Model file for the job. Use its own axes, mm. Face numbers are marked on the shaded views. A direction names the side the tool comes from. Coordinates: 2 decimals unless noted, no trailing zeros. Write each loop counter-clockwise with the first axis right and the second up, starting at its lowest first coordinate (ties: lowest second). Pieces come first, ordered by that corner, then holes. Notation, with made-up numbers: (4, 31.5) -> (8, 31.5) arc R36 cw to (8, 66.5) -> close; hole circle Ø6 at (41, 73.5). An arc over 180 degrees is marked (long way). Write item = value, one per line. Start each with the question number.
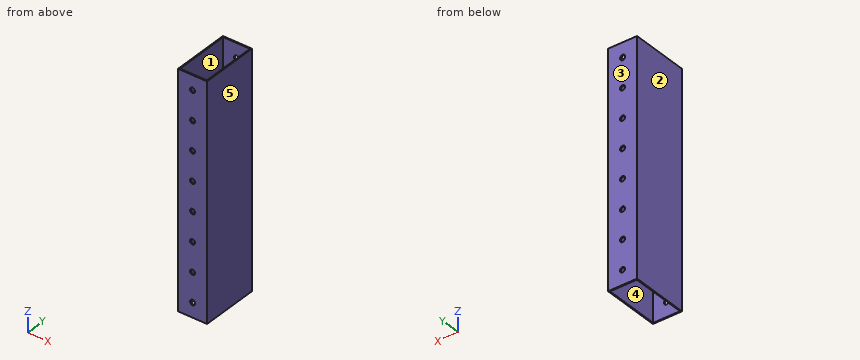
Autodesk Inventor part; units mm, degrees
ref_plane "YZ Plane" through (0, 0, 0) normal (1, 0, 0) x (0, 1, 0)
ref_plane "XZ Plane" through (0, 0, 0) normal (0, 1, 0) x (-1, 0, 0)
ref_plane "XY Plane" through (0, 0, 0) normal (0, 0, 1) x (1, 0, 0)
sketch "Sketch1" plane through (0, 0, 0) normal (0, 0, 1) x (1, 0, 0)
  line L0 (12.7, 25.4) -> (-12.7, 25.4)
  line L1 (-12.7, 25.4) -> (-12.7, -25.4)
  line L2 (-12.7, -25.4) -> (12.7, -25.4)
  line L3 (12.7, -25.4) -> (12.7, 25.4)
  line L4 (12.7, 25.4) -> (-12.7, -25.4) construction
  line L5 (-12.7, 25.4) -> (12.7, -25.4) construction
  line L6 (-11.684, 24.384) -> (11.684, 24.384)
  line L7 (11.684, 24.384) -> (11.684, -24.384)
  line L8 (11.684, -24.384) -> (-11.684, -24.384)
  line L9 (-11.684, -24.384) -> (-11.684, 24.384)
  point P0 (0, 0)
  dimension "d0" = 1.016
  dimension "d1" = 50.8
  dimension "d2" = 25.4
extrude "Tube Length" add sketch "Sketch1" along normal mid plane 203.2
sketch "Sketch2" plane through (-12.7, 25.4, 101.6) normal (0, 1, 0) x (1, 0, 0)
  line L0 (0, 0) -> (0, 203.2)
  line L1 (25.4, 0) -> (0, 0)
  line L2 (25.4, 203.2) -> (25.4, 0)
  line L3 (0, 203.2) -> (25.4, 203.2)
  line L4 (25.4, 0) -> (0, 0)
  line L5 (12.7, 0) -> (12.7, 12.7) construction
  circle A0 centre (12.7, 12.7) radius 2.2479
  point P0 (12.7, 101.6)
  dimension "d5" = 12.7
  dimension "d6" = 4.4958
extrude "Top Hole" cut sketch "Sketch2" against normal through all contours A0
pattern_linear "Rectangular Pattern1" count 8 spacing 25.4 along (0, 0, -1) of "Top Hole"
sketch "Sketch3" plane through (0, 0, 101.6) normal (0, 0, 1) x (1, 0, 0)
  line L0 (0, 0) -> (0, 25.4) construction
  line L1 (12.7, 25.4) -> (-12.7, 25.4)
  line L2 (-0.0508, 25.4) -> (0, 25.2984)
  line L3 (0.0508, 25.4) -> (0, 25.2984)
  line L4 (-12.7, 12.6492) -> (-12.5984, 12.7)
  line L5 (-12.7, 12.7508) -> (-12.5984, 12.7)
  line L6 (-12.7, -0.0508) -> (-12.5984, 0)
  line L7 (-12.7, 0.0508) -> (-12.5984, 0)
  line L8 (-12.7, -12.7508) -> (-12.5984, -12.7)
  line L9 (-12.7, -12.6492) -> (-12.5984, -12.7)
  line L10 (12.7, 0.0508) -> (12.5984, 0)
  line L11 (12.7, 12.6492) -> (12.5984, 12.7)
  line L12 (12.7, 12.7508) -> (12.5984, 12.7)
  line L13 (12.7, -0.0508) -> (12.5984, 0)
  line L14 (12.7, -12.6492) -> (12.5984, -12.7)
  line L15 (12.7, -12.7508) -> (12.5984, -12.7)
  line L16 (0.0508, -25.4) -> (0, -25.2984)
  line L17 (-0.0508, -25.4) -> (0, -25.2984)
  line L18 (-12.7, 25.4) -> (-12.7, -25.4)
  line L19 (12.7, -25.4) -> (12.7, 25.4)
  line L20 (-12.7, -25.4) -> (12.7, -25.4)
  point P0 (0, 12.7)
  point P1 (-12.7, 12.7)
  point P2 (-12.7, 0)
  point P3 (-12.7, -12.7)
  point P4 (12.7, 12.7)
  point P5 (12.7, 0)
  point P6 (12.7, -12.7)
  point P7 (0, -25.4)
  dimension "d12" = 0.1016
  dimension "d13" = 0.1016
  dimension "d16" = 90
  dimension "d20" = 12.7
  dimension "d27" = 360
equation "\"d13\" = d12"
properties part number "Carrage Side Tube" material "Aluminum 6061"
(1) Drop a flat-ended pin along its axis: pin 1 Ø4 at (x, z) = (0, 12.7) entering from +Y. Give the stop position or say it passes through.
(2) Saw through at C-C (x = 8.5). Give the cut face in (y, z), then the cut area to 3 significant figures.
(3) Saw through at B-B (y = 1). Give the cut face in (x, z), then the cut area to 3 significant figures.
(4) Mould opens along Y. For the marked faces 1, 2 and 3 say: released by +Y, released by -Y, zero draft, split by the parting line, or undercut.
(5) 3-axis set-ups, long thin cutter, end or side, ignore diameter. For the marked faces 4 and 5: which of +Z, -Z, +X, -X, +Y, -Y reach the whole face in a straight line?
(6) Drill centre lines: line 1 along X through (y, z) = (24.6, 63.5); line 2 along Y through (x, z) = (11.25, -86); line 3 along X through (y, z) = (7, 28). Where is each one in solid material? Low to high.
(7) Saw through at A-A (z = -63.5). Give the cut face in (x, y).
(8) Saw through at D-D (x = 0). State how many separate pieces and enclosed holes the cut face has, then the cut area to 3 significant figures.
Returned:
q1.pin_1 = through
q2.outline = (-25.4, -101.6) -> (-24.38, -101.6) -> (-24.38, 101.6) -> (-25.4, 101.6) -> close; (24.38, -101.6) -> (25.4, -101.6) -> (25.4, 101.6) -> (24.38, 101.6) -> close
q2.area = 413 mm2
q3.outline = (-12.7, -101.6) -> (-11.68, -101.6) -> (-11.68, 101.6) -> (-12.7, 101.6) -> close; (11.68, -101.6) -> (12.7, -101.6) -> (12.7, 101.6) -> (11.68, 101.6) -> close
q3.area = 413 mm2
q4.face_1 = undercut
q4.face_2 = zero draft
q4.face_3 = released by +Y
q5.face_4 = +Z, -Z
q5.face_5 = +Z, -Z, +X, +Y, -Y
q6.line_1 = -12.7 to -2.25, 2.25 to 12.7
q6.line_2 = -25.4 to -24.38, 24.38 to 25.4
q6.line_3 = -12.7 to -11.68, 11.68 to 12.7
q7.outline = (-12.7, -25.4) -> (-2.25, -25.4) -> (-2.25, -24.38) -> (-11.68, -24.38) -> (-11.68, 24.38) -> (-2.25, 24.38) -> (-2.25, 25.4) -> (-12.7, 25.4) -> close; (2.25, -25.4) -> (12.7, -25.4) -> (12.7, 25.4) -> (2.25, 25.4) -> (2.25, 24.38) -> (11.68, 24.38) -> (11.68, -24.38) -> (2.25, -24.38) -> close
q8.separate_pieces = 18
q8.enclosed_holes = 0
q8.area = 340 mm2
